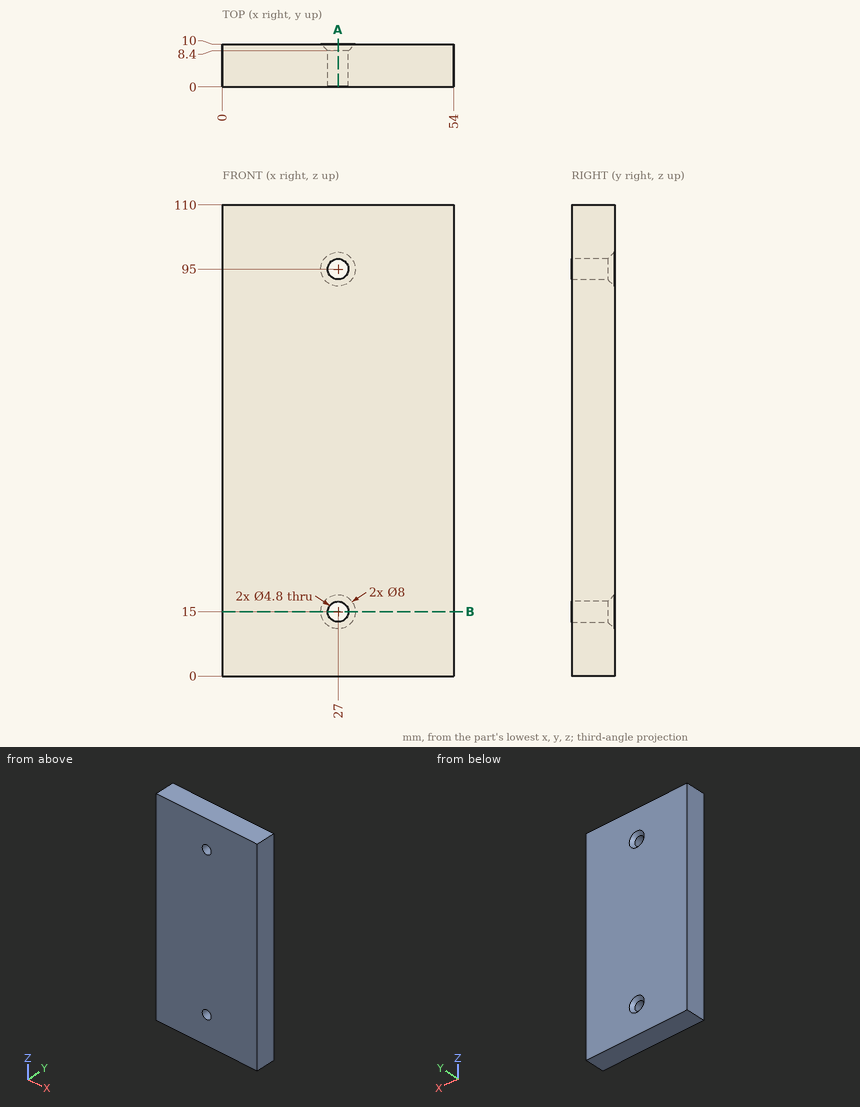
Design review of the part shown in the three views and the two pictorial views. Dimensions are in mm from the part's minimum x, y and z. Round coordinates to 2 decimals unless told otherwise and drop trailing zeros. Order: outer loops, then holes, each group sorted by start corner. A loop starts at its lowest first (then second) coordinate and runs counter-clockwise, first axis right, second up. Notation, with made-up numbers: (40.5, 6) - (69.5, 6) arc R14 ccw to (69.5, 31) - close; hole circle Ø9 at (58.5, 3.5). An arc over 180 degrees is marked (long way). Answer in a Markdown table with one row per item.
(1) For line 1 (X direction, y = 4.5, z = 15); line 2 (X direction, y = 7, z = 93), list the stretches that pass through material, from the lowest coordinate up. Write a range as from..to.
Result set:
| item | result |
|---|---|
| line 1 | x = 0..24.6, 29.4..54 |
| line 2 | x = 0..25.67, 28.33..54 |
(2) Clearance check with a flat-ended pin moving along its axis: P1, Ø7.5, axis at x = 27, z = 15, coming from the +Y side. State where the tip first meets the part, or that it passes through.
Result set:
| item | result |
|---|---|
| P1 | stops at y = 9.75 |
(3) Take a section at A-A on x = 27. Write out the cut boundary in (y, z), plus the area to 3 significant figures.
Result set:
| item | result |
|---|---|
| outline | (0, 0) - (10, 0) - (10, 11) - (8.4, 12.6) - (0, 12.6) - close; (0, 17.4) - (8.4, 17.4) - (10, 19) - (10, 91) - (8.4, 92.6) - (0, 92.6) - close; (0, 97.4) - (8.4, 97.4) - (10, 99) - (10, 110) - (0, 110) - close |
| area | 999 mm2 |
(4) Take a section at B-B on z = 15. Write out the cut boundary in (x, y), plus the area to 3 significant figures.
Result set:
| item | result |
|---|---|
| outline | (0, 0) - (24.6, 0) - (24.6, 8.4) - (23, 10) - (0, 10) - close; (29.4, 0) - (54, 0) - (54, 10) - (31, 10) - (29.4, 8.4) - close |
| area | 489 mm2 |
